Check sheet for the modelled part. Datum: model origin and axes. Units: mm. Round coordinates to 2 decimals unless told otherwise and drop trailing zeros. Loops run counter-clockwise (first coordinate to the right, second up) from the corner with the lowest first, then second, coordinate; pieces in that order, holes last. Notation, with made-up numbers: (68, 65.25) - (77, 65.25) arc R15 cw to (77, 85.25) - close; hole circle Ø6 at (87, 85). An arc over 180 degrees is marked (long way). Put each result on its own line as item: value.
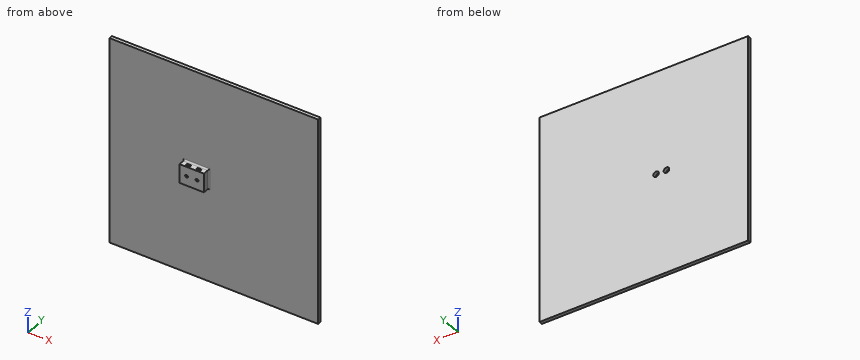
Autodesk Inventor part; units mm, degrees
ref_plane "YZ Plane" through (0, 0, 0) normal (1, 0, 0) x (0, 1, 0)
ref_plane "XZ Plane" through (0, 0, 0) normal (0, 1, 0) x (-1, 0, 0)
ref_plane "XY Plane" through (0, 0, 0) normal (0, 0, 1) x (1, 0, 0)
sketch "Sketch1" plane through (0, 0, 0) normal (0, 1, 0) x (-1, 0, 0)
  line L0 (-150, 150) -> (150, 150)
  line L1 (150, 150) -> (150, -150)
  line L2 (150, -150) -> (-150, -150)
  line L3 (-150, -150) -> (-150, 150)
  line L4 (-150, 150) -> (150, -150) construction
  line L5 (150, 150) -> (-150, -150) construction
  line L6 (150, 0) -> (-150, 0) construction
  line L7 (0, 150) -> (0, -150) construction
  line L8 (37.5, 6.35) -> (-37.5, 6.35) construction
  line L9 (-37.5, 6.35) -> (-37.5, -6.35) construction
  line L10 (-37.5, -6.35) -> (37.5, -6.35) construction
  line L11 (37.5, -6.35) -> (37.5, 6.35) construction
  line L12 (37.5, 6.35) -> (-37.5, -6.35) construction
  line L13 (-37.5, 6.35) -> (37.5, -6.35) construction
  circle A0 centre (32.5, 0) radius 2
  circle A1 centre (17.5, 0) radius 2
  circle A2 centre (-32.5, 0) radius 2 construction
  circle A3 centre (-17.5, 0) radius 2 construction
  line L14 (30.5, 0) -> (19.5, 0) construction
  line L15 (42.5, 13.75) -> (7.5, 13.75)
  line L16 (7.5, 13.75) -> (7.5, -13.75)
  line L17 (7.5, -13.75) -> (42.5, -13.75)
  line L18 (42.5, -13.75) -> (42.5, 13.75)
  line L19 (42.5, 13.75) -> (7.5, -13.75) construction
  line L20 (7.5, 13.75) -> (42.5, -13.75) construction
  circle A4 centre (32.5, 0) radius 4
  circle A5 centre (17.5, 0) radius 4
  point P0 (0, 0)
  point P1 (37.5, 0)
  point P2 (25, 0)
  dimension "d4" = 4
  dimension "d7" = 4
  dimension "d0" = 300
  dimension "d1" = 300
  dimension "d2" = 75
  dimension "d3" = 12.7
  dimension "d5" = 5
  dimension "d8" = 15
  dimension "d9" = 35
  dimension "d10" = 27.5
  dimension "d15" = 8
  dimension "d16" = 8
extrude "Extrusion1" add sketch "Sketch1" along normal blind 5 contours L0 L1 L2 L3 | L18 L17 L16 L15 | A4 | A5
extrude "Extrusion2" add sketch "Sketch1" against normal blind 10 contours L18 L17 L16 L15 | A4 | A5
extrude "Extrusion3" cut sketch "Sketch1" along normal blind 10 contours A4 | A5
fillet "Fillet1" radius 2 4 edges at (-42.5, 0, 0) (-25, 0, 13.75) (-25, 0, -13.75) (-7.5, 0, 0)
sketch "Sketch2" plane through (-42.5, -10, 13.75) normal (0, 0, 1) x (1, 0, 0)
  line L0 (0, 8) -> (35, 8)
  line L1 (0, 8) -> (0, 0)
  line L2 (35, 0) -> (0, 0)
  line L3 (35, 8) -> (35, 0)
  line L4 (10, 8) -> (10, 0) construction
  line L5 (7, 5.6) -> (13, 5.6)
  line L6 (13, 5.6) -> (13, 2.4)
  line L7 (13, 2.4) -> (7, 2.4)
  line L8 (7, 2.4) -> (7, 5.6)
  line L9 (7, 5.6) -> (13, 2.4) construction
  line L10 (13, 5.6) -> (7, 2.4) construction
  line L11 (0, 4) -> (10, 4) construction
  line L12 (35, 0) -> (0, 0)
  line L13 (17.5, 0) -> (17.5, 8) construction
  line L14 (28, 5.6) -> (22, 5.6)
  line L15 (22, 5.6) -> (22, 2.4)
  line L16 (22, 2.4) -> (28, 2.4)
  line L17 (28, 2.4) -> (28, 5.6)
  line L18 (28, 5.6) -> (22, 2.4) construction
  line L19 (22, 5.6) -> (28, 2.4) construction
  point P0 (42.5, 10)
  point P1 (25, 4)
  dimension "d20" = 10
  dimension "d21" = 6
  dimension "d22" = 3.2
extrude "Extrusion4" cut sketch "Sketch2" against normal blind 16.75 contours L5 L6 L7 L8 | L17 L16 L15 L14
properties part number "PlataformaLoadCell" material "PC/ABS Plastic"
Item 1: Go/stop test with flat-tipped pins: pin 1 (4 mm diameter, centred on y = -7, z = 0.5, fed in from +X); pin 2 (1 mm diameter, centred on y = -6, z = 1.5, fed in from -X); pin 3 (3.5 mm diameter, centred on x = -31.5, y = -6.5, fed in from +Z); pin 4 (2.5 mm diameter, centred on x = -32.5, z = 0, fed in from +Y). Record where each tip stops, or that it passes through.
Filled sheet:
pin 1: x = -7.5
pin 2: x = -42.5
pin 3: z = 13.75
pin 4: through
Item 2: Thickness scan on line 1 (X direction, y = 2.55, z = 0); line 2 (X direction, y = -4.75, z = 9); line 3 (Z direction, x = -17.5, y = 1.9). Record the ranges inside material, lowest first. Write a range as from..to.
Filled sheet:
line 1: -150..-36.5, -28.5..-21.5, -13.5..150
line 2: -42.5..-35.5, -29.5..-20.5, -14.5..-7.5
line 3: -150..-4, 4..150
Item 3: Section check C-C on x = -110. Enter the section's corners in (y, z).
Filled sheet:
outline: (0, -150) - (5, -150) - (5, 150) - (0, 150) - close
Item 4: Section check B-B on z = 111. Enter the section's corners in (x, y), then the cut area to 3 significant figures.
Filled sheet:
outline: (-150, 0) - (150, 0) - (150, 5) - (-150, 5) - close
area: 1,500 mm²
Item 5: Section check A-A on z = 10. Enter the section's corners in (x, y).
Filled sheet:
outline: (-150, 0) - (-44.5, 0) arc R2 cw to (-42.5, -2) - (-42.5, -10) - (-7.5, -10) - (-7.5, -2) arc R2 cw to (-5.5, 0) - (150, 0) - (150, 5) - (-150, 5) - close; hole (-35.5, -7.6) - (-29.5, -7.6) - (-29.5, -4.4) - (-35.5, -4.4) - close; hole (-20.5, -7.6) - (-14.5, -7.6) - (-14.5, -4.4) - (-20.5, -4.4) - close
